from build123d import *

# Parameters (mm, degrees)
SKETCH1_W               = 5
SKETCH1_H               = 5
SKETCH1_W_2             = 4.9
SKETCH1_H_2             = 4
BOSS_EXTRUDE1_DEPTH     = 41.1
CUT_EXTRUDE1_DEPTH      = 42.478428128
CUT_EXTRUDE1_DEPTH_BACK = 0.05
SKETCH2_W               = 2.5
SKETCH2_H               = 2.5


with BuildPart() as part:
    # Sketch1 → Boss-Extrude1 (new body)
    with BuildSketch(Plane(origin=(0, 0, 0), x_dir=(1, 0, 0), z_dir=(0, 1, 0))):
        Rectangle(SKETCH1_W, SKETCH1_H)
        Rectangle(SKETCH1_W_2, SKETCH1_H_2, mode=Mode.SUBTRACT)
    extrude(amount=BOSS_EXTRUDE1_DEPTH)

    # Sketch2 → Cut-Extrude1 (cut, two sides: drawn at the far end of the back side and taken through both)
    with BuildSketch(Plane.ZY.offset(2.5).offset(-CUT_EXTRUDE1_DEPTH_BACK)):
        with Locations((0, 2.25)):
            Rectangle(SKETCH2_W, SKETCH2_H)
    extrude(amount=CUT_EXTRUDE1_DEPTH + CUT_EXTRUDE1_DEPTH_BACK, mode=Mode.SUBTRACT)


solid = part.part
Check sheet for the modelled part. Datum: model origin and axes. Units: mm. Coordinates: 2 decimals unless noted, no trailing zeros. Write each loop counter-clockwise with the first axis right and the second up, starting at its lowest first coordinate (ties: lowest second). Pieces come first, ordered by that corner, then holes.
Item 1: Cross-section at B-B on x = 0.1. Record the boundary of the cut face in (y, z).
Numbers:
outline: (0, -2.5) - (41.1, -2.5) - (41.1, -2) - (0, -2) - close; (0, 2) - (41.1, 2) - (41.1, 2.5) - (0, 2.5) - close
Item 2: Depth check by flat-ended pin: pin 1 Ø3 at (x, z) = (1, -0.5) entering from -Y. Enter the tip coordinate at first touch or a pass-through.
Numbers:
pin 1: stops at y = 0
Item 3: Mould release check, pull along Z, two halves, no side actions. Record for faces 1 (the face through (0, 20, -2.5)), 2 (the face through (0, 20, 2.5)), 3 (the face through (0, 20, -2)): released by +Z, released by -Z, zero draft, split by the parting line, or undercut.
Numbers:
face 1: released by -Z
face 2: released by +Z
face 3: undercut
Item 4: Scan line: probe 1 along Z at (x, y) = (-0.6, 36). Record every from-to range of solid material in increasing order.
Numbers:
probe 1: z = -2.5 to -2, 2 to 2.5
Item 5: Cross-section at C-C on y = 19. Record the boundary of the cut face in (x, z).
Numbers:
outline: (-2.5, -2.5) - (2.5, -2.5) - (2.5, 2.5) - (-2.5, 2.5) - close; hole (-2.45, -2) - (2.45, -2) - (2.45, 2) - (-2.45, 2) - close
Item 6: Cross-section at A-A on z = 0.5. Record the boundary of the cut face in (x, y).
Numbers:
outline: (-2.5, 0) - (-2.45, 0) - (-2.45, 1) - (-2.5, 1) - close; (-2.5, 3.5) - (-2.45, 3.5) - (-2.45, 41.1) - (-2.5, 41.1) - close; (2.45, 0) - (2.5, 0) - (2.5, 41.1) - (2.45, 41.1) - close
